Could you check a few things on this model? Use its own coordinates, in mm. A direction names the side the tool comes from. Round coordinates to 2 decimals unless told otherwise and drop trailing zeros. Loops run counter-clockwise (first coordinate to the right, second up) from the corner with the lowest first, then second, coordinate; pieces in that order, holes last. Notation, with made-up numbers: (-13.5, -34.75) - (24.5, -34.75) arc R13 ccw to (24.5, -19.75) - close; hole circle Ø11 at (59.25, 68.25). An arc over 180 degrees is marked (long way). Answer as CSV lines item,"result". Start each with the question number.
1) We'd pull the mould along X, two halves only. Please class faces 1 (the face through (10.336, 7, 118)), 2 (the face through (0, -4, 118)), 3 (the face through (-4, 0, 118)), 4 (the face through (7, 10.336, 118)): pulls with the +X half, pulls with the -X half, needs draft (parallel to the pull), parting line crosses it, or undercut.
2) I'm going to push flat-ended pins straight in: pin 1 Ø4.5 at (x, z) = (0, 121) entering from -Y; pin 2 Ø6 at (y, z) = (0.5, 114.5) entering from +X; pin 3 Ø3 at (x, y) = (0.5, -7.5) entering from +Z. Where does each tip first touch, or does it pass through?
3) Suppose I cut it at A-A, the plane y = 0. Write out the boundary of the cut face in (x, z), then the cut area to 3 significant figures.
4) Please list where these lines run through material, in increasing order: line 1 along Y through (x, z) = (-0.25, 137); line 2 along Y through (x, z) = (6.25, 101); line 3 along X through (y, z) = (4.5, 21).
5) Which directions (+Z, -Z, +X, -X, +Y, -Y) give clear straight access to the entire face, cutting with the end or side of a thin tool? Please do faces 5 (the face through (4, 0, 118)), 6 (the face through (-0.54, -2.44, 118.32)), 7 (the face through (0, 4, 118)).
```python
from build123d import *

# Parameters (mm, degrees)
SKETCH2_R           = 2.5
BOSS_EXTRUDE2_DEPTH = 240


with BuildPart() as part:
    # Sketch2 → Boss-Extrude2 (new body)
    with BuildSketch(Plane.XY):
        with BuildLine():
            Line((-10.33624689, -3.6), (-10.33624689, -10.33624689))
            Line((-10.33624689, -10.33624689), (-3.1, -10.33624689))
            Line((-3.1, -10.33624689), (-3.1, -8.33624689))
            Line((-3.1, -8.33624689), (-5.990764132, -8.33624689))
            ThreePointArc((-5.990764132, -8.33624689), (-6.545144596, -7.965729571), (-6.414833183, -7.311787894))
            Line((-6.414833183, -7.311787894), (-3.392837365, -4.29256834))
            ThreePointArc((-3.392837365, -4.29256834), (-3.068526748, -4.07603256), (-2.686055612, -4))
            Line((-2.686055612, -4), (2.686055612, -4))
            ThreePointArc((2.686055612, -4), (3.068526748, -4.07603256), (3.392837365, -4.29256834))
            Line((3.392837365, -4.29256834), (6.414833183, -7.311787894))
            ThreePointArc((6.414833183, -7.311787894), (6.545144596, -7.965729571), (5.990764132, -8.33624689))
            Line((5.990764132, -8.33624689), (3.1, -8.33624689))
            Line((3.1, -8.33624689), (3.1, -10.33624689))
            Line((3.1, -10.33624689), (10.33624689, -10.33624689))
            Line((10.33624689, -10.33624689), (10.33624689, -3.6))
            Line((10.33624689, -3.6), (9.83624689, -3.6))
            Line((9.83624689, -3.6), (9.83624689, -3.1))
            Line((9.83624689, -3.1), (8.33624689, -3.1))
            Line((8.33624689, -3.1), (8.33624689, -5.99013487))
            ThreePointArc((8.33624689, -5.99013487), (7.965755883, -6.544504441), (7.31182815, -6.414244211))
            Line((7.31182815, -6.414244211), (4.292635434, -3.392848919))
            ThreePointArc((4.292635434, -3.392848919), (4.076050714, -3.068515006), (4, -2.686000016))
            Line((4, -2.686000016), (4, 2.686000016))
            ThreePointArc((4, 2.686000016), (4.076050714, 3.068515006), (4.292635434, 3.392848919))
            Line((4.292635434, 3.392848919), (7.31182815, 6.414244211))
            ThreePointArc((7.31182815, 6.414244211), (7.965755883, 6.544504441), (8.33624689, 5.99013487))
            Line((8.33624689, 5.99013487), (8.33624689, 3.1))
            Line((8.33624689, 3.1), (9.83624689, 3.1))
            Line((9.83624689, 3.1), (9.83624689, 3.6))
            Line((9.83624689, 3.6), (10.33624689, 3.6))
            Line((10.33624689, 3.6), (10.33624689, 10.33624689))
            Line((10.33624689, 10.33624689), (3.1, 10.33624689))
            Line((3.1, 10.33624689), (3.1, 8.33624689))
            Line((3.1, 8.33624689), (5.990764132, 8.33624689))
            ThreePointArc((5.990764132, 8.33624689), (6.545144596, 7.965729571), (6.414833183, 7.311787894))
            Line((6.414833183, 7.311787894), (3.392837365, 4.29256834))
            ThreePointArc((3.392837365, 4.29256834), (3.068526748, 4.07603256), (2.686055612, 4))
            Line((2.686055612, 4), (-2.686055612, 4))
            ThreePointArc((-2.686055612, 4), (-3.068526748, 4.07603256), (-3.392837365, 4.29256834))
            Line((-3.392837365, 4.29256834), (-6.414833183, 7.311787894))
            ThreePointArc((-6.414833183, 7.311787894), (-6.545144596, 7.965729571), (-5.990764132, 8.33624689))
            Line((-5.990764132, 8.33624689), (-3.1, 8.33624689))
            Line((-3.1, 8.33624689), (-3.1, 10.33624689))
            Line((-3.1, 10.33624689), (-10.33624689, 10.33624689))
            Line((-10.33624689, 10.33624689), (-10.33624689, 3.6))
            Line((-10.33624689, 3.6), (-9.83624689, 3.6))
            Line((-9.83624689, 3.6), (-9.83624689, 3.1))
            Line((-9.83624689, 3.1), (-8.33624689, 3.1))
            Line((-8.33624689, 3.1), (-8.33624689, 5.99013487))
            ThreePointArc((-8.33624689, 5.99013487), (-7.965755883, 6.544504441), (-7.31182815, 6.414244211))
            Line((-7.31182815, 6.414244211), (-4.292635434, 3.392848919))
            ThreePointArc((-4.292635434, 3.392848919), (-4.076050714, 3.068515006), (-4, 2.686000016))
            Line((-4, 2.686000016), (-4, -2.686000016))
            ThreePointArc((-4, -2.686000016), (-4.076050714, -3.068515006), (-4.292635434, -3.392848919))
            Line((-4.292635434, -3.392848919), (-7.31182815, -6.414244211))
            ThreePointArc((-7.31182815, -6.414244211), (-7.965755883, -6.544504441), (-8.33624689, -5.99013487))
            Line((-8.33624689, -5.99013487), (-8.33624689, -3.1))
            Line((-8.33624689, -3.1), (-9.83624689, -3.1))
            Line((-9.83624689, -3.1), (-9.83624689, -3.6))
            Line((-9.83624689, -3.6), (-10.33624689, -3.6))
        make_face()
        Circle(SKETCH2_R, mode=Mode.SUBTRACT)
    extrude(amount=BOSS_EXTRUDE2_DEPTH)


solid = part.part
```
Filled sheet:
1,face 1,"pulls with the +X half"
1,face 2,"undercut"
1,face 3,"pulls with the -X half"
1,face 4,"needs draft"
2,pin 1,"y = -4"
2,pin 2,"x = 9.84"
2,pin 3,"through"
3,outline,"(-4, 0) - (-2.5, 0) - (-2.5, 240) - (-4, 240) - close; (2.5, 0) - (4, 0) - (4, 240) - (2.5, 240) - close"
3,area,"720 mm²"
4,line 1,"-4 to -2.49, 2.49 to 4"
4,line 2,"-10.34 to -8.28, -7.15 to -5.35, 5.35 to 7.15, 8.28 to 10.34"
4,line 3,"-10.34 to -8.34, -5.4 to -3.6, 3.6 to 5.4, 8.34 to 10.34"
5,face 5,"+Z, -Z, +X"
5,face 6,"+Z, -Z"
5,face 7,"+Z, -Z, +Y"
